The listing builds one solid part. Answer for the finished solid, in the listing's coordinates (mm). Round coordinates to 2 decimals unless told otherwise and drop trailing zeros. Write each loop counter-clockwise with the first axis right and the second up, starting at its lowest first coordinate (ties: lowest second). Pieces come first, ordered by that corner, then holes.
Item 1: Find the intervals of material crossed by probe 1 along Y at (x, z) = (40, 2); probe 2 along Y at (x, z) = (-40, 1.85); probe 3 along X at (y, z) = (25, 3.25), in increasing order.
Item 2: Find section B-B on y = 25. Give the number of separate pieces and of enclosed holes in the cut face, then the cut area to 3 significant figures.
Item 3: Find section A-A on x = 13. Give the vertices of the cut face in (y, z).
Item 4: This flat-tipped pin is pushed along its axis until it touches: pin 1 (4 mm diameter, centred on x = 40, y = -25, fed in from -Z). Where does it stop, or does it pass through?
Autodesk Inventor part; units mm, degrees
ref_plane "YZ Plane" through (0, 0, 0) normal (1, 0, 0) x (0, 1, 0)
ref_plane "XZ Plane" through (0, 0, 0) normal (0, 1, 0) x (-1, 0, 0)
ref_plane "XY Plane" through (0, 0, 0) normal (0, 0, 1) x (1, 0, 0)
sketch "Sketch1" plane through (0, 0, 0) normal (0, 0, 1) x (1, 0, 0)
  line L0 (-50, -35) -> (50, -35)
  line L1 (50, -35) -> (50, 35)
  line L2 (50, 35) -> (-50, 35)
  line L3 (-50, 35) -> (-50, -35)
  line L4 (-50, -35) -> (50, 35) construction
  line L5 (50, -35) -> (-50, 35) construction
  point P0 (0, 0)
  dimension "d0" = 100
  dimension "d1" = 70
extrude "Extrusion1" add sketch "Sketch1" along normal blind 3.5
sketch "Sketch2" plane through (0, 0, 3.5) normal (0, 0, 1) x (1, 0, 0)
  circle A0 centre (-40, 25) radius 2.3
  line L0 (-70, 0) -> (70, 0)
  line L1 (0, -49) -> (0, 49)
  circle A1 centre (40, 25) radius 2.3
  circle A2 centre (-40, -25) radius 2.3
  circle A3 centre (40, -25) radius 2.3
  point P0 (0, 0)
  dimension "d4" = 40
  dimension "d5" = 25
  dimension "d6" = 4.6
extrude "Extrusion2" cut sketch "Sketch2" against normal up to surface (3.5 mm away)
fillet "Fillet1" radius 15 4 edges at (-50, 35, 1.75) (-50, -35, 1.75) (50, -35, 1.75) (50, 35, 1.75)
chamfer "Chamfer2" distance 0.5 angle 45 12 edges at (-50, 0, 0) (-45.6066, -30.6066, 0) (0, -35, 0) (45.6066, -30.6066, 0) (50, 0, 0) (45.6066, 30.6066, 0) (0, 35, 0) (-45.6066, 30.6066, 0) (-42.3, -25, 0) (-42.3, 25, 0) (37.7, 25, 0) (37.7, -25, 0)
chamfer "Chamfer3" distance 0.5 angle 45 4 edges at (-42.3, 25, 3.5) (37.7, 25, 3.5) (37.7, -25, 3.5) (-42.3, -25, 3.5)
chamfer "Chamfer4" distance 2 angle 45 8 edges at (-50, 0, 3.5) (-45.6066, -30.6066, 3.5) (0, -35, 3.5) (45.6066, -30.6066, 3.5) (50, 0, 3.5) (45.6066, 30.6066, 3.5) (0, 35, 3.5) (-45.6066, 30.6066, 3.5)
properties part number "_3DPrint"
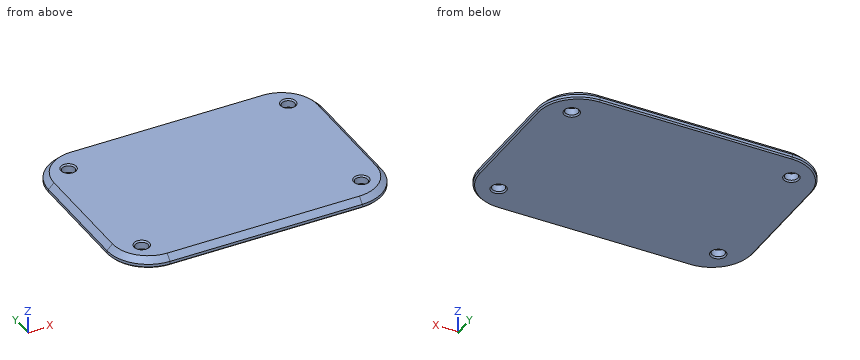
Check values:
1. probe 1: y = -33.61 to -27.3, -22.7 to 22.7, 27.3 to 33.61
1. probe 2: y = -33.77 to -27.3, -22.7 to 22.7, 27.3 to 33.77
1. probe 3: x = -47.27 to -42.55, -37.45 to 37.45, 42.55 to 47.27
2. separate pieces: 3
2. enclosed holes: 0
2. area: 306 mm2
3. outline: (-35, 0.5) - (-34.5, 0) - (34.5, 0) - (35, 0.5) - (35, 1.5) - (33, 3.5) - (-33, 3.5) - (-35, 1.5) - close
4. pin 1: passes through
